Geometry check sheet. Reference: the model listing, model coordinates, mm. A direction names the side the tool comes from. Coordinates: 2 decimals unless noted, no trailing zeros. Order: outer loops, then holes, each group sorted by start corner. A loop starts at its lowest first (then second) coordinate and runs counter-clockwise, first axis right, second up. Notation, with made-up numbers: (41.5, 83) - (93.5, 83) arc R25 ccw to (93.5, 114) - close; hole circle Ø8 at (47, -26). An arc over 180 degrees is marked (long way). Return JSON: item names as keys, results as strings. Group by question number.
Item 1: Gauge pin test, flat ends, axial feed: pin 1 (2 mm diameter, centred on y = 13, z = 33.5, fed in from -X); pin 2 (1 mm diameter, centred on y = -10, z = 136, fed in from +X); pin 3 (6 mm diameter, centred on x = 8.5, z = 118, fed in from +Y). Record the tip position at first contact, or that the pin passes through.
Item 2: Section check D-D on z = 67. Enter the section's corners in (x, y) (3 decimals).
Item 3: Scan lines: probe 1 along Z at (x, y) = (12.5, -9); probe 2 along X at (y, z) = (-1.5, 143); probe 3 along X at (y, z) = (6, 136.5). Record each from-to range of solid material in increasing order.
Item 4: Tool access check on faces 1 (the flat face through (15.875, 0, 47)), 2 (the flat face through (0, 0, 112.268)). Record the directions out of +Z, -Z, +X, -X, +Y, -Y that give a thin tool (end or side, any length) a straight path to the whole face; none if there is none.
Item 5: Draft check along Y on faces 3 (the flat face through (-3.131, 5.525, 132.615)), 4 (the flat face through (0, 0, 19.05)), 5 (the flat face through (-8.049, -13.684, 47.225)), 6 (the flat face through (-3.219, -5.474, 132.615)). Enter one of: pulls with the +Y half, pulls with the -Y half, needs draft (parallel to the pull), parting line crosses it, or undercut.
Item 6: Section check B-B on z = 51.5. Enter the section's corners in (x, y) (3 decimals).
Item 7: Section check C-C on z = 129. Enter the section's corners in (x, y).
Item 8: Section check A-A on y = 0. Enter the section's corners in (x, z) (3 decimals).
from build123d import *

# Parameters (mm, degrees)
BOSS_EXTRUDE1_DEPTH      = 152.4
BOSS_EXTRUDE1_DEPTH_BACK = 152.4
CUT_EXTRUDE1_DEPTH       = 171.45
CUT_EXTRUDE2_DEPTH       = 40.132
SKETCH6_R                = 18.330871047
SKETCH6_R_2              = 12.7
CUT_EXTRUDE3_DEPTH       = 76.2
SKETCH7_R                = 6.35
CUT_EXTRUDE4_DEPTH       = 157.747705991


with BuildPart() as part:
    # Sketch3 → Boss-Extrude1 (new, two sides: drawn at the far end of the back side and taken through both)
    with BuildSketch(Plane.XY.offset(-BOSS_EXTRUDE1_DEPTH_BACK)):
        Polygon((0, 18.330871047), (-15.875, 9.165435523), (-15.875, -9.165435523), (0, -18.330871047), (15.875, -9.165435523), (15.875, 9.165435523), align=None)
    extrude(amount=BOSS_EXTRUDE1_DEPTH + BOSS_EXTRUDE1_DEPTH_BACK)

    # Sketch4 → Cut-Extrude1 (cut)
    with BuildSketch(Plane(origin=(0, 0, -152.4), x_dir=(-1, 0, 0), z_dir=(0, 0, -1))):
        Polygon((0, 18.330871047), (-15.875, 9.165435523), (-15.875, -9.165435523), (0, -18.330871047), (15.875, -9.165435523), (15.875, 9.165435523), align=None)
    extrude(amount=-CUT_EXTRUDE1_DEPTH, mode=Mode.SUBTRACT)

    # Sketch5 → Cut-Extrude2 (cut)
    with BuildSketch(Plane.XY.offset(152.4)):
        Polygon((0, 7.332348419), (-6.35, 3.666174209), (-6.35, -3.666174209), (0, -7.332348419), (6.35, -3.666174209), (6.35, 3.666174209), align=None)
    extrude(amount=-CUT_EXTRUDE2_DEPTH, mode=Mode.SUBTRACT)

    # Sketch6 → Cut-Extrude3 (cut)
    with BuildSketch(Plane.XY.offset(152.4)):
        Circle(SKETCH6_R)
        Circle(SKETCH6_R_2, mode=Mode.SUBTRACT)
    extrude(amount=-CUT_EXTRUDE3_DEPTH, mode=Mode.SUBTRACT)

    # Sketch7 → Cut-Extrude4 (cut, through all)
    with BuildSketch(Plane(origin=(15.875, 0, 0), x_dir=(0, 0, -1), z_dir=(1, 0, 0))):
        with Locations((-53.594, 0)):
            Circle(SKETCH7_R)
    extrude(amount=-CUT_EXTRUDE4_DEPTH, mode=Mode.SUBTRACT)


solid = part.part
Computed:
{
 "1": {"pin 1": "stops at x = -10.97", "pin 2": "stops at x = 8.43", "pin 3": "stops at y = 11.45"},
 "2": {"outline": "(-15.875, -9.165) - (0, -18.331) - (15.875, -9.165) - (15.875, 9.165) - (0, 18.331) - (-15.875, 9.165) - close"},
 "3": {"probe 1": "z = 19.05 to 76.2", "probe 2": "x = -12.61 to -6.35, 6.35 to 12.61", "probe 3": "x = -11.19 to -2.31, 2.31 to 11.19"},
 "4": {"face 1": "+Z, -Z, +X, +Y, -Y", "face 2": "+Z"},
 "5": {"face 3": "undercut", "face 4": "needs draft", "face 5": "pulls with the -Y half", "face 6": "undercut"},
 "6": {"outline": "(-15.875, -9.165) - (0, -18.331) - (15.875, -9.165) - (15.875, -5.995) - (-15.875, -5.995) - close; (-15.875, 5.995) - (15.875, 5.995) - (15.875, 9.165) - (0, 18.331) - (-15.875, 9.165) - close"},
 "7": {"outline": "circle Ø25.4 at (0, 0); hole (-6.35, -3.67) - (0, -7.33) - (6.35, -3.67) - (6.35, 3.67) - (0, 7.33) - (-6.35, 3.67) - close"},
 "8": {"outline": "(-15.875, 19.05) - (15.875, 19.05) - (15.875, 47.244) - (-15.875, 47.244) - close; (-15.875, 59.944) - (15.875, 59.944) - (15.875, 76.2) - (12.7, 76.2) - (12.7, 152.4) - (6.35, 152.4) - (6.35, 112.268) - (-6.35, 112.268) - (-6.35, 152.4) - (-12.7, 152.4) - (-12.7, 76.2) - (-15.875, 76.2) - close"}
}
